```python
from build123d import *

# Parameters (mm, degrees)
BOSS_EXTRUDE1_DEPTH      = 1.5875
BOSS_EXTRUDE1_DEPTH_BACK = 1.5875
SKETCH3_R                = 3.571875


with BuildPart() as part:
    # Sketch3 → Boss-Extrude1 (new, two sides: drawn at the far end of the back side and taken through both)
    with BuildSketch(Plane.XY.offset(-BOSS_EXTRUDE1_DEPTH_BACK)):
        Polygon((-10.31875, -23.8125), (10.31875, -23.8125), (10.31875, 3.175), (37.30625, 3.175), (37.30625, 23.8125), (-37.30625, 23.8125), (-37.30625, 3.175), (-10.31875, 3.175), align=None)
        with Locations((26.9875, 13.49375)):
            Circle(SKETCH3_R, mode=Mode.SUBTRACT)
        with Locations((0, -13.49375)):
            Circle(SKETCH3_R, mode=Mode.SUBTRACT)
        with Locations((-26.9875, 13.49375)):
            Circle(SKETCH3_R, mode=Mode.SUBTRACT)
        with Locations((0, 13.49375)):
            Circle(SKETCH3_R, mode=Mode.SUBTRACT)
    extrude(amount=BOSS_EXTRUDE1_DEPTH + BOSS_EXTRUDE1_DEPTH_BACK)


solid = part.part
```
Design review of the part built by this model. Coordinates are the model's own, in mm. A direction names the side the tool comes from. Coordinates: 2 decimals unless noted, no trailing zeros. Order: outer loops, then holes, each group sorted by start corner. A loop starts at its lowest first (then second) coordinate and runs counter-clockwise, first axis right, second up. Notation, with made-up numbers: (36.25, 65) -> (45.25, 65) arc R8 cw to (45.25, 80) -> close; hole circle Ø11 at (6.25, 1.5). An arc over 180 degrees is marked (long way). One line per item, written item: value. Start each with the question number.
Q1. Mouldability with a two-part tool opening along X and no side actions: class faces 4 (the flat face through (-10.319, -10, 0)), 5 (the flat face through (0, -23.812, 0)), 6 (the cylindrical face through (-30.556, 13.651, -0.022)) as pulls with the +X half, pulls with the -X half, needs draft (parallel to the pull), parting line crosses it, or undercut.
Q2. Take a section at D-D, the plane x = -22. State the section outline as (y, z) points (1 decimal).
Q3. Tool access review of faces 1 (the flat face through (24, 3.175, 0)), 2 (the flat face through (1, 23.812, 0)), 3 (the flat face through (-24, 3.175, 0)): name each direction out of +Z, -Z, +X, -X, +Y, -Y from which nothing blocks a thin tool from reaching the whole face with its end or side.
Q4. Take a section at C-C, the plane y = -16. State the section outline as (x, z) points (1 decimal).
Q5. Take a section at B-B, the plane z = -0.7. State the section outline as (x, y) points (1 decimal), then the cut area to 3 significant figures.
Q6. Insertion check: pin 1 Ø1 at (x, z) = (10.5, -0.5) entering from -Y; pin 2 Ø1.6 at (y, z) = (-7, -0.5) entering from -X; pin 3 Ø1 at (y, z) = (-10.5, 0) entering from +X. Each pin has a flat end and moves straight along its axis. Give the tip position at first contact, or say it passes through.
Q7. For probe 1 along Y at (x, z) = (0, -0.3); probe 2 along Y at (x, z) = (-2, -0.4); probe 3 along X at (y, z) = (10.5, -0.8), list the stretches that pass through material, from the lowest coordinate up.
Q8. Take a section at A-A, the plane x = 0. State the section outline as (y, z) points.
Values follow:
1. face 4: pulls with the -X half
1. face 5: needs draft
1. face 6: undercut
2. outline: (3.2, -1.6) -> (23.8, -1.6) -> (23.8, 1.6) -> (3.2, 1.6) -> close
3. face 1: +Z, -Z, +X, -Y
3. face 2: +Z, -Z, +X, -X, +Y
3. face 3: +Z, -Z, -X, -Y
4. outline: (-10.3, -1.6) -> (-2.5, -1.6) -> (-2.5, 1.6) -> (-10.3, 1.6) -> close; (2.5, -1.6) -> (10.3, -1.6) -> (10.3, 1.6) -> (2.5, 1.6) -> close
5. outline: (-37.3, 3.2) -> (-10.3, 3.2) -> (-10.3, -23.8) -> (10.3, -23.8) -> (10.3, 3.2) -> (37.3, 3.2) -> (37.3, 23.8) -> (-37.3, 23.8) -> close; hole circle Ø7.1 at (-27, 13.5); hole circle Ø7.1 at (0, -13.5); hole circle Ø7.1 at (0, 13.5); hole circle Ø7.1 at (27, 13.5)
5. area: 1,940 mm2
6. pin 1: stops at y = -23.81
6. pin 2: stops at x = -10.32
6. pin 3: stops at x = 10.32
7. probe 1: y = -23.81 to -17.07, -9.92 to 9.92, 17.07 to 23.81
7. probe 2: y = -23.81 to -16.45, -10.53 to 10.53, 16.45 to 23.81
7. probe 3: x = -37.31 to -28.94, -25.04 to -1.95, 1.95 to 25.04, 28.94 to 37.31
8. outline: (-23.81, -1.59) -> (-17.07, -1.59) -> (-17.07, 1.59) -> (-23.81, 1.59) -> close; (-9.92, -1.59) -> (9.92, -1.59) -> (9.92, 1.59) -> (-9.92, 1.59) -> close; (17.07, -1.59) -> (23.81, -1.59) -> (23.81, 1.59) -> (17.07, 1.59) -> close
